from build123d import *

# Parameters (mm, degrees)
F0_R     = 2.5
F1_DEPTH = 3.5
F2_DEPTH = 60
F3_SIZE  = 1
F4_SIZE  = 0.2


with BuildPart() as f1:
    # F0 (on Top) → F1 (new body)
    with BuildSketch(Plane.XY):
        Polygon((2.280534, 3.95), (-2.280534, 3.95), (-4.561067, 0), (-2.280534, -3.95), (2.280534, -3.95), (4.561067, 0), align=None)
        Circle(F0_R, mode=Mode.SUBTRACT)
        Circle(F0_R)
    extrude(amount=F1_DEPTH)

    # F0 (on Top) → F2 (join)
    with BuildSketch(Plane.XY):
        Circle(F0_R)
    extrude(amount=-F2_DEPTH)

    # F3
    f3_edges = [f1.edges().sort_by_distance(p)[0] for p in [
        (-2.5, 0, -60),
    ]]
    chamfer(f3_edges, length=F3_SIZE)

    # F4
    f4_edges = [f1.edges().sort_by_distance(p)[0] for p in [
        (0, 3.95, 3.5),
        (-3.4208, 1.975, 3.5),
        (-3.4208, -1.975, 3.5),
        (0, -3.95, 3.5),
        (3.4208, -1.975, 3.5),
        (3.4208, 1.975, 3.5),
        (0, 3.95, 0),
        (3.4208, 1.975, 0),
        (-3.4208, 1.975, 0),
        (3.4208, -1.975, 0),
        (-3.4208, -1.975, 0),
        (0, -3.95, 0),
        (-2.5, 0, 0),
    ]]
    chamfer(f4_edges, length=F4_SIZE)


solid = f1.part
Here's how the part is built. I have some questions about the finished solid (model axes, mm). A direction names the side the tool comes from. Round coordinates to 2 decimals unless told otherwise and drop trailing zeros. Order: outer loops, then holes, each group sorted by start corner. A loop starts at its lowest first (then second) coordinate and runs counter-clockwise, first axis right, second up. Notation, with made-up numbers: M 3.25,-13 L 27.25,-13 A16 ccw 27.25,-8 Z; hole C 9.5,29.25 d4. An arc over 180 degrees is marked long. Return JSON: item names as keys, results as strings. Group by question number.
1. If we section it at B-B on z = -51: List the corners of the cut face in (x, y) for me.
2. On a 3-axis mill with a long thin cutter (end or side, diameter ignored), from which of +Z, -Z, +X, -X, +Y, -Y can I reach the whole of each face in a straight line? I mean faces 4 (the face through (-3.405, 2.003, 1.728)), 5 (the face through (-0.54, -2.44, -29.19)). Say none if no direction works.
3. I'm going to push flat-ended pins straight in: pin 1 Ø4 at (x, z) = (3.5, -3.5) entering from +Y; pin 2 Ø3 at (x, z) = (2.5, -49) entering from +Y; pin 3 Ø2 at (y, z) = (-1, -18) entering from -X. Where does each tip first touch, or does it pass through?
4. If we section it at A-A on x = 0: List the corners of the cut face in (y, z) for me.
5. If we mould it in two halves opening along Z, with no side actions, what happens to faces 1 (the face through (1, 3, 0)), 2 (the face through (0, 0, 3.5)), 3 (the face through (3.405, -2.003, 1.728))? For each: pulls with the +Z half, pulls with the -Z half, needs draft (parallel to the pull), parting line crosses it, or undercut.
6. Please list where these lines run through material, in increasing order: probe 1 along Z at (x, y) = (2.75, 2.25); probe 2 along X at (y, z) = (-1, -5.5); probe 3 along Y at (x, z) = (2, -10.5).
Reply:
{
 "1": {"outline": "C 0,0 d5"},
 "2": {"face 4": "+Z, -Z, -X, +Y", "face 5": "-Z"},
 "3": {"pin 1": "y = 2", "pin 2": "y = 2.29", "pin 3": "x = -2.5"},
 "4": {"outline": "M -3.95,0.2 L -3.75,0 L -2.7,0 L -2.5,-0.2 L -2.5,-59 L -1.5,-60 L 1.5,-60 L 2.5,-59 L 2.5,-0.2 L 2.7,0 L 3.75,0 L 3.95,0.2 L 3.95,3.3 L 3.75,3.5 L -3.75,3.5 L -3.95,3.3 Z"},
 "5": {"face 1": "pulls with the -Z half", "face 2": "pulls with the +Z half", "face 3": "needs draft"},
 "6": {"probe 1": "0 to 3.5", "probe 2": "-2.29 to 2.29", "probe 3": "-1.5 to 1.5"}
}
